Geometry check sheet. Reference: the model listing, model coordinates, mm. A direction names the side the tool comes from. Coordinates: 2 decimals unless noted, no trailing zeros. Write each loop counter-clockwise with the first axis right and the second up, starting at its lowest first coordinate (ties: lowest second). Pieces come first, ordered by that corner, then holes. Notation, with made-up numbers: M -16.75,28.25 L 2.25,28.25 A13 cw 2.25,32.25 Z; hole C 88,63 d9. An arc over 180 degrees is marked long. Write item = value, one per line. Start each with the question number.
Autodesk Inventor part; units mm, degrees
ref_plane "YZ Plane" through (0, 0, 0) normal (1, 0, 0) x (0, 1, 0)
ref_plane "XZ Plane" through (0, 0, 0) normal (0, 1, 0) x (-1, 0, 0)
ref_plane "XY Plane" through (0, 0, 0) normal (0, 0, 1) x (1, 0, 0)
sketch "Эскиз1" plane through (0, 0, 0) normal (0, 0, 1) x (1, 0, 0)
  circle A0 centre (0, 0) radius 1.5
  circle A1 centre (0, 0) radius 2.75
  dimension "d0" = 5.5
  dimension "d1" = 3
extrude "Выдавливание1" add sketch "Эскиз1" along normal blind 16 contours A0
extrude "Выдавливание2" add sketch "Эскиз1" against normal blind 1.5 contours A0 | A1
thread "Резьба1"
sketch "Эскиз2" plane through (0, 0, -1.5) normal (0, 0, -1) x (-1, 0, 0)
  line L0 (0, 1.1547) -> (1, 0.5774)
  line L1 (1, 0.5774) -> (1, -0.5774)
  line L2 (1, -0.5774) -> (0, -1.1547)
  line L3 (0, -1.1547) -> (-1, -0.5774)
  line L4 (-1, -0.5774) -> (-1, 0.5774)
  line L5 (-1, 0.5774) -> (0, 1.1547)
  point P0 (0, 0)
  point P1 (0, 0)
  dimension "d8" = 2
extrude "Выдавливание3" cut sketch "Эскиз2" against normal blind 1
fillet "Сопряжение1" radius 1 1 edges at (-2.75, 0, -1.5)
properties part number "Болт М3 16 мм"
Q1. Cross-section at A-A on y = 0. Enter the section's corners in (x, z), and give its area (3 significant figures).
Q2. Gauge pin test, flat ends, axial feed: pin 1 (0.5 mm diameter, centred on y = 0, z = -1, fed in from -X); pin 2 (1 mm diameter, centred on x = 1.5, y = -1, fed in from +Z); pin 3 (1.5 mm diameter, centred on y = 0.5, z = 6, fed in from +X). Record the tip position at first contact, or that the pin passes through.
Q3. Scan lines: L1, parallel to Z at x = 1.6, y = -0.7; L2, parallel to Z at x = 0.35, y = -0.4; L3, parallel to X at y = -0.1, z = 8.5. Record each from-to range of solid material in increasing order.
Q4. Draft check along Y on faces 4 (the face through (-1, 0, -1)), 5 (the face through (-1.5, -0.07, 7.89)), 6 (the face through (0, 0, 16)). Enter one of: pulls with the +Y half, pulls with the -Y half, needs draft (parallel to the pull), parting line crosses it, or undercut.
Q5. Cross-section at B-B on z = 1. Enter the section's corners in (x, y).
Q6. Set-up check for faces 1 (the face through (1, -1, -1.5)), 2 (the face through (0.51, 0.86, -1.01)), 3 (the face through (1.2, -1.2, 0)): record each of +Z, -Z, +X, -X, +Y, -Y from which the full face is reachable in a straight line by a thin tool's end or side.
Values found:
q1.outline = M -2.75,-0.5 A1 ccw -1.75,-1.5 L -1,-1.5 L -1,-0.5 L 1,-0.5 L 1,-1.5 L 1.75,-1.5 A1 ccw 2.75,-0.5 L 2.75,0 L 1.5,0 L 1.5,16 L -1.5,16 L -1.5,0 L -2.75,0 Z
q1.area = 53.8 mm²
q2.pin_1 = -2.72
q2.pin_2 = 16
q2.pin_3 = 1.5
q3.L1 = -1.5 to 0
q3.L2 = -0.5 to 16
q3.L3 = -1.5 to 1.5
q4.face_4 = undercut
q4.face_5 = parting line crosses it
q4.face_6 = needs draft
q5.outline = C 0,0 d3
q6.face_1 = -Z, +X, -X, +Y, -Y
q6.face_2 = -Z
q6.face_3 = +Z
